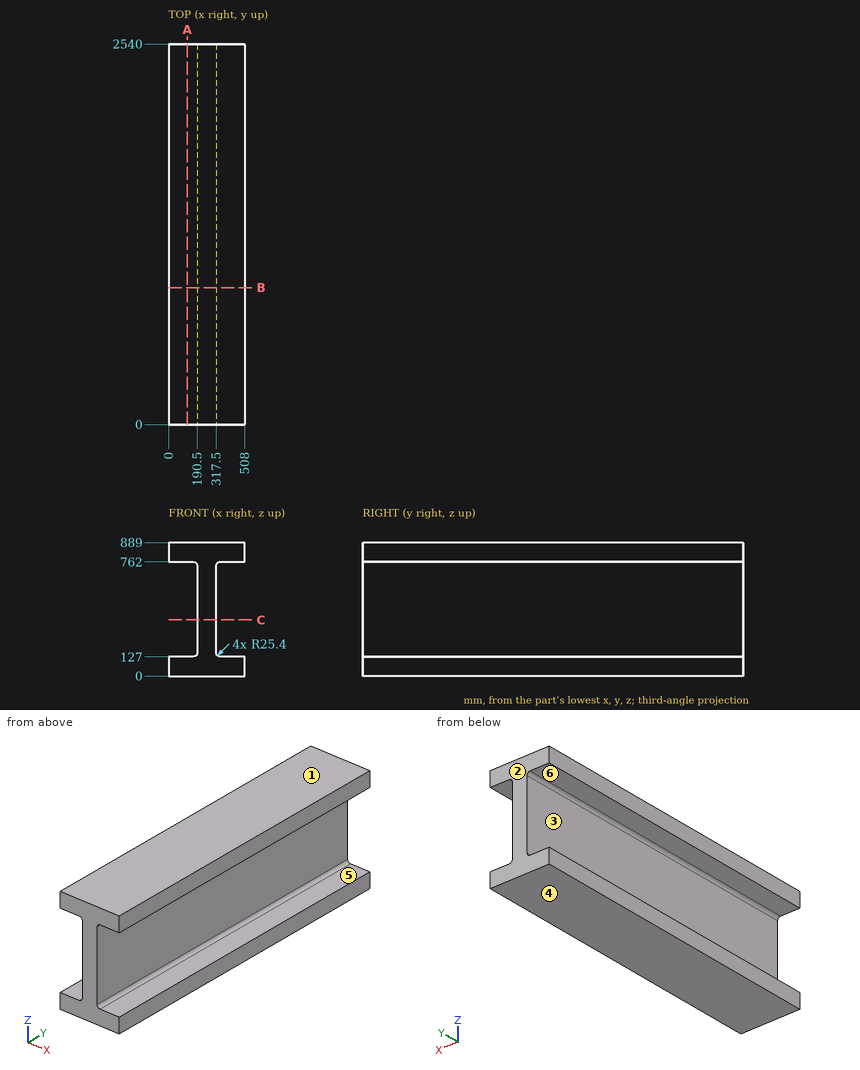
Design review of the part shown in the three views and the two pictorial views. Dimensions are in mm from the part's minimum x, y and z. A direction names the side the tool comes from. Round coordinates to 2 decimals unless told otherwise and drop trailing zeros. Write each loop counter-clockwise with the first axis right and the second up, starting at its lowest first coordinate (ties: lowest second). Pieces come first, ordered by that corner, then holes. Notation, with made-up numbers: (-4.5, -5) - (11.5, -5) arc R22 ccw to (11.5, 23) - close; hole circle Ø8 at (25.25, -32). An arc over 180 degrees is marked (long way). Answer as CSV lines item,"result". Start each with the question number.
(1) Mouldability with a two-part tool opening along Z and no side actions: class the marked faces 1, 2 and 3 as +Z half, -Z half, draft (parallel to the pull), parting line (faces both ways), or undercut.
(2) Machinability: for the marked faces 4, 5 and 6, which of the approach directions +Z, -Z, +X, -X, +Y, -Y give a long, thin tool a straight path to every point of the face, cutting with its end or side? Answer none if there is none.
(3) For pin 1 (6 mm diameter, centred on y = 1872.5, z = 442.5, fed in from -X), flat-tipped, find the tip position at first contact; note if it passes through.
(4) Add section C-C, the plane z = 374. State the section outline as (x, y) points.
(5) Add section A-A, the plane x = 125. State the section outline as (y, z) points, plus the area to 3 significant figures.
(6) For line 1 (Z direction, x = 105, y = 2175); line 2 (X direction, y = 1636, z = 193.5), list the stretches that pass through material, from the lowest coordinate up.
(7) Add section B-B, the plane y = 915. State the section outline as (x, z) points.
From the geometry:
1,face 1,"+Z half"
1,face 2,"draft"
1,face 3,"undercut"
2,face 4,"-Z, +X, -X, +Y, -Y"
2,face 5,"+X, +Y, -Y"
2,face 6,"-X, +Y, -Y"
3,pin 1,"stops at x = 190.5"
4,outline,"(190.5, 0) - (317.5, 0) - (317.5, 2540) - (190.5, 2540) - close"
5,outline,"(0, 0) - (2540, 0) - (2540, 127) - (0, 127) - close; (0, 762) - (2540, 762) - (2540, 889) - (0, 889) - close"
5,area,"645,000 mm²"
6,line 1,"z = 0 to 127, 762 to 889"
6,line 2,"x = 190.5 to 317.5"
7,outline,"(0, 0) - (508, 0) - (508, 127) - (342.9, 127) arc R25.4 cw to (317.5, 152.4) - (317.5, 736.6) arc R25.4 cw to (342.9, 762) - (508, 762) - (508, 889) - (0, 889) - (0, 762) - (165.1, 762) arc R25.4 cw to (190.5, 736.6) - (190.5, 152.4) arc R25.4 cw to (165.1, 127) - (0, 127) - close"
